The listing builds one solid part. Answer for the finished solid, in the listing's coordinates (mm). Give positions to 0.01 mm unless a question says otherwise; leave off trailing zeros. Write each loop counter-clockwise with the first axis right and the second up, starting at its lowest first coordinate (ties: lowest second). Pieces come first, ordered by that corner, then holes. Notation, with made-up numbers: (57.25, -39.75) - (67.25, -39.75) arc R25 ccw to (67.25, -9.75) - close; hole circle Ø10 at (36, -32). An arc over 180 degrees is marked (long way). Return JSON: item names as keys, results as strings.
from build123d import *

# Parameters (mm, degrees)
F0_W     = 42
F0_H     = 42
F0_R     = 2
F0_R_2   = 11.05
F1_DEPTH = 4
F2_SIZE  = 5
F3_SIZE  = 5
F4_SIZE  = 5
F5_SIZE  = 5


with BuildPart() as f1:
    # F0 (on Front) → F1 (new body)
    with BuildSketch(Plane.XZ):
        Rectangle(F0_W, F0_H)
        with Locations((-15, -15)):
            Circle(F0_R, mode=Mode.SUBTRACT)
        with Locations((15, -15)):
            Circle(F0_R, mode=Mode.SUBTRACT)
        with Locations((-15, 15)):
            Circle(F0_R, mode=Mode.SUBTRACT)
        Circle(F0_R_2, mode=Mode.SUBTRACT)
        with Locations((15, 15)):
            Circle(F0_R, mode=Mode.SUBTRACT)
    extrude(amount=F1_DEPTH)

    # F2
    f2_edges = [f1.edges().sort_by_distance(p)[0] for p in [
        (-21, -2, -21),
    ]]
    chamfer(f2_edges, length=F2_SIZE)

    # F3
    f3_edges = [f1.edges().sort_by_distance(p)[0] for p in [
        (-21, -2, 21),
    ]]
    chamfer(f3_edges, length=F3_SIZE)

    # F4
    f4_edges = [f1.edges().sort_by_distance(p)[0] for p in [
        (21, -2, 21),
    ]]
    chamfer(f4_edges, length=F4_SIZE)

    # F5
    f5_edges = [f1.edges().sort_by_distance(p)[0] for p in [
        (21, -2, -21),
    ]]
    chamfer(f5_edges, length=F5_SIZE)


solid = f1.part
Item 1: Flat-ended cylindrical pins translate along their axes: P1, Ø13.5, axis at x = 0, z = 0, coming from the +Y side; P2, Ø4.5, axis at x = 15, z = 15, coming from the +Y side. Find the tip coordinate at first contact, or state that the pin passes through.
Answer below:
{"P1": "passes through", "P2": "stops at y = 0"}
Item 2: Consider L1, parallel to Z at x = 15, y = -1.65; L2, parallel to X at y = -2.65, z = -14.5; L3, parallel to X at y = -3.25, z = -13.5. Determine where each line is inside the solid, lowest interval first.
Answer below:
{"L1": "z = -21 to -17, -13 to 13, 17 to 21", "L2": "x = -21 to -16.94, -13.06 to 13.06, 16.94 to 21", "L3": "x = -21 to -16.32, -13.68 to 13.68, 16.32 to 21"}
Item 3: A cutting plane is placed at C-C on z = -15. Determine the outline of the cut face in (x, y).
Answer below:
{"outline": "(-21, -4) - (-17, -4) - (-17, 0) - (-21, 0) - close; (-13, -4) - (13, -4) - (13, 0) - (-13, 0) - close; (17, -4) - (21, -4) - (21, 0) - (17, 0) - close"}
Item 4: A cutting plane is placed at B-B on x = 0. Determine the outline of the cut face in (y, z).
Answer below:
{"outline": "(-4, -21) - (0, -21) - (0, -11.05) - (-4, -11.05) - close; (-4, 11.05) - (0, 11.05) - (0, 21) - (-4, 21) - close"}
Item 5: A cutting plane is placed at A-A on z = 0. Determine the outline of the cut face in (x, y), then the cut area to 3 significant figures.
Answer below:
{"outline": "(-21, -4) - (-11.05, -4) - (-11.05, 0) - (-21, 0) - close; (11.05, -4) - (21, -4) - (21, 0) - (11.05, 0) - close", "area": "79.6 mm²"}
Item 6: The mould has two halves that part along X. Classify faces 1 (the face through (-21, -2, 0)), 2 (the face through (15, -2, 17)), 3 (the face through (0, -2, -21)): +X half, -X half, draft (parallel to the pull), parting line (faces both ways), or undercut.
Answer below:
{"face 1": "-X half", "face 2": "undercut", "face 3": "draft"}
Item 7: A cutting plane is placed at D-D on x = -15. Determine the outline of the cut face in (y, z).
Answer below:
{"outline": "(-4, -21) - (0, -21) - (0, -17) - (-4, -17) - close; (-4, -13) - (0, -13) - (0, 13) - (-4, 13) - close; (-4, 17) - (0, 17) - (0, 21) - (-4, 21) - close"}
